from build123d import *

# Parameters (mm, degrees)
BOSS_EXTRUDE1_DEPTH = 210
BOSS_EXTRUDE2_START = 210
BOSS_EXTRUDE2_DEPTH = 10
BOSS_EXTRUDE3_START = -210
BOSS_EXTRUDE3_DEPTH = 10


with BuildPart() as part:
    # Sketch1 → Boss-Extrude1 (new body, symmetric)
    with BuildSketch(Plane.XY):
        with BuildLine():
            Line((-134.629120178, 10), (-125, 10))
            Line((-125, 10), (-125, 0))
            ThreePointArc((-125, 0), (0, -125), (125, 0))
            Line((125, 0), (125, 10))
            Line((125, 10), (134.629120178, 10))
            ThreePointArc((134.629120178, 10), (0, -135), (-134.629120178, 10))
        make_face()
    extrude(amount=BOSS_EXTRUDE1_DEPTH, both=True)

    # Sketch2 → Boss-Extrude2 (add)
    with BuildSketch(Plane.XY.offset(BOSS_EXTRUDE2_START)):
        with BuildLine():
            Line((-125, 10), (-12, 10))
            ThreePointArc((-12, 10), (0, -2), (12, 10))
            Line((12, 10), (125, 10))
            Line((125, 10), (125, 0))
            ThreePointArc((125, 0), (0, -125), (-125, 0))
            Line((-125, 0), (-125, 10))
        make_face()
    extrude(amount=-BOSS_EXTRUDE2_DEPTH)

    # Sketch2<2> → Boss-Extrude3 (add)
    with BuildSketch(Plane.XY.offset(BOSS_EXTRUDE3_START)):
        with BuildLine():
            Line((-12, 10), (-125, 10))
            Line((-125, 10), (-125, 0))
            ThreePointArc((-125, 0), (0, -125), (125, 0))
            Line((125, 0), (125, 10))
            Line((125, 10), (12, 10))
            ThreePointArc((12, 10), (0, -2), (-12, 10))
        make_face()
        with BuildLine():
            Line((-125, 0), (-125, 10))
            Line((-125, 10), (-134.629120178, 10))
            ThreePointArc((-134.629120178, 10), (0, -135), (134.629120178, 10))
            Line((134.629120178, 10), (125, 10))
            Line((125, 10), (125, 0))
            ThreePointArc((125, 0), (0, -125), (-125, 0))
        make_face()
    extrude(amount=BOSS_EXTRUDE3_DEPTH)


solid = part.part
Work out the finished part from the listing and answer in its coordinate system (mm). A direction names the side the tool comes from. Coordinates: 2 decimals unless noted, no trailing zeros. Loops run counter-clockwise (first coordinate to the right, second up) from the corner with the lowest first, then second, coordinate; pieces in that order, holes last. Notation, with made-up numbers: M -21,67.25 L 20,67.25 A31 ccw 20,91.25 Z; hole C 73.25,23.25 d6. An arc over 180 degrees is marked long. Answer in a Markdown table with one row per item. Add a question column.
1. The mould has two halves that part along X. Classify faces 1 (the cylindrical face through (0, -2, 205)), 2 (the flat face through (-2, -45, -210)), 3 (the flat face through (2, -42, 200)), 4 (the cylindrical face through (3.109, -134.964, 2.94)): pulls with the +X half, pulls with the -X half, needs draft (parallel to the pull), parting line crosses it, or undercut.
2. Consider L1, parallel to Z at x = 30, y = -103.5; L2, parallel to Y at x = 4, z = 95.5; L3, parallel to X at y = -92.5, z = -24.5. Determine where each line is inside the solid, lowest interval first.
3. A tool of negligible diameter and unlimited length cuts with its end or side. For faces 5 (the flat face through (-125, 5, 3)), 6 (the flat face through (2, -45, 210)), from which of +Z, -Z, +X, -X, +Y, -Y can it reach the whole face along a straight path? Write none if from no direction.
4. Find section D-D, the plane y = -47.5. Write down the section's boundary in (x, z), then the cut area to 3 significant figures.
5. Find section B-B, the plane x = 0. Write down the section's boundary in (y, z).
6. Find section A-A, the plane y = -103.5. Write down the section's boundary in (x, z).
7. Find section C-C, the plane z = 14. Write down the section's boundary in (x, y), then the cut area to 3 significant figures.
8. Flat-ended cylindrical pins translate along their axes: P1, Ø2, axis at y = -99, z = -79.5, coming from the +X side; P2, Ø3, axis at x = 9, z = 167.5, coming from the -Y side; P3, Ø4, axis at y = -57, z = 6.5, coming from the -X side. Find the tip coordinate at first contact, or state that the pin passes through.
Reported:
| question | item | result |
|---|---|---|
| 1 | face 1 | undercut |
| 1 | face 2 | needs draft |
| 1 | face 3 | undercut |
| 1 | face 4 | parting line crosses it |
| 2 | L1 | z = -210 to -200, 200 to 210 |
| 2 | L2 | y = -134.94 to -124.94 |
| 2 | L3 | x = -98.33 to -84.08, 84.08 to 98.33 |
| 3 | face 5 | +Y |
| 3 | face 6 | +Z, +X, -X, +Y, -Y |
| 4 | outline | M -126.37,-210 L 126.37,-210 L 126.37,210 L -126.37,210 Z; hole M -115.62,-200 L 115.62,-200 L 115.62,200 L -115.62,200 Z |
| 4 | area | 13,700 mm^2 |
| 5 | outline | M -135,-210 L -2,-210 L -2,-200 L -125,-200 L -125,200 L -2,200 L -2,210 L -135,210 Z |
| 6 | outline | M -86.68,-210 L 86.68,-210 L 86.68,210 L -86.68,210 Z; hole M -70.09,-200 L 70.09,-200 L 70.09,200 L -70.09,200 Z |
| 7 | outline | M -134.63,10 A135 ccw long 134.63,10 L 125,10 L 125,0 A125 cw -125,0 L -125,10 Z |
| 7 | area | 4,280 mm^2 |
| 8 | P1 | stops at x = 92.85 |
| 8 | P2 | stops at y = -134.79 |
| 8 | P3 | stops at x = -123.29 |
